Input: dimensioned drawing with shaded views. Units: mm. Origin: part minimum x, y, z. A direction names the side the tool comes from. Coordinates: 2 decimals unless noted, no trailing zeros. Write each loop counter-clockwise with the first axis right and the second up, starting at its lowest first coordinate (ties: lowest second). Pieces come first, ordered by that corner, then holes. Notation, with made-up numbers: M 85.5,-17.5 L 124.5,-17.5 A10 ccw 124.5,0.5 Z; hole C -15,60.5 d9. An arc over 180 degrees is marked long. Use one line per item in the form item = value.
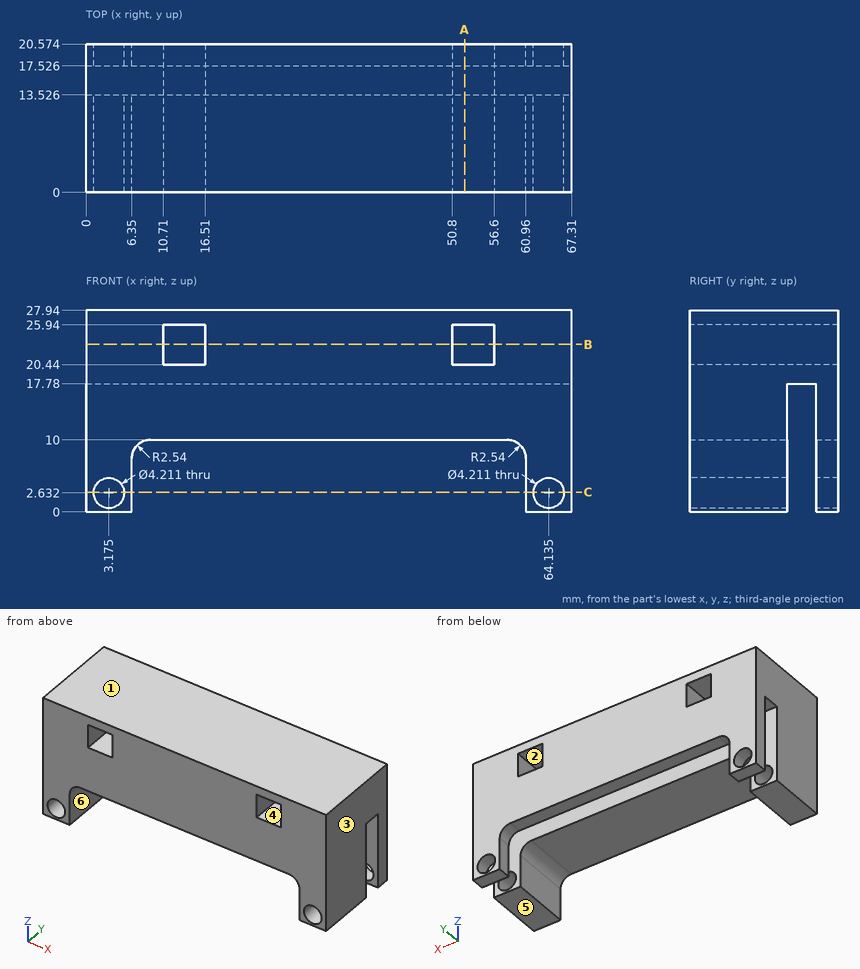
(1) Pull-direction query (X, two-part tool) for the marked faces 1, 2 and 3; classes: pulls with the +X half, pulls with the -X half, needs draft (parallel to the pull), parting line crosses it, or undercut.
Computed:
face_1 = needs draft
face_2 = undercut
face_3 = pulls with the +X half
(2) Line query: probe 1 along X at (y, z) = (10, 23.25); probe 2 along Y at (x, z) = (33, 16.25); probe 3 along X at (y, z) = (9.5, 6.75). Output: solid intervals per line, ascending.
Computed:
probe_1 = 0 to 10.71, 16.51 to 50.8, 56.6 to 67.31
probe_2 = 0 to 13.53, 17.53 to 20.57
probe_3 = 0 to 6.35, 60.96 to 67.31
(3) Set-up query: the marked faces 4, 5 and 6. Return all of +Z, -Z, +X, -X, +Y, -Y with unobstructed straight access to the full face (end or side cutting, diameter ignored); none if empty.
Computed:
face_4 = +Y, -Y
face_5 = -Z, +X, -X, +Y, -Y
face_6 = -Z, +Y, -Y
(4) Section query C-C on z = 2.75. State how many separate pieces and enclosed holes the cut face has.
Computed:
separate_pieces = 8
enclosed_holes = 0
(5) First-contact query: pin 1 Ø12 at (x, y) = (41, 8.5) entering from -Z. Flat tip, straight axial feed; report the tip coordinate or a pass-through.
Computed:
pin_1 = 10
(6) Section query B-B on z = 23.25. Return the cut outline in (x, y).
Computed:
outline = M 0,0 L 10.71,0 L 10.71,20.57 L 0,20.57 Z; M 16.51,0 L 50.8,0 L 50.8,20.57 L 16.51,20.57 Z; M 56.6,0 L 67.31,0 L 67.31,20.57 L 56.6,20.57 Z
(7) Section query A-A on x = 52.5. Return the cut outline in (y, z), plus the area to 3 significant figures.
Computed:
outline = M 0,10 L 13.53,10 L 13.53,17.78 L 17.53,17.78 L 17.53,10 L 20.57,10 L 20.57,20.44 L 0,20.44 Z; M 0,25.94 L 20.57,25.94 L 20.57,27.94 L 0,27.94 Z
area = 225 mm^2
